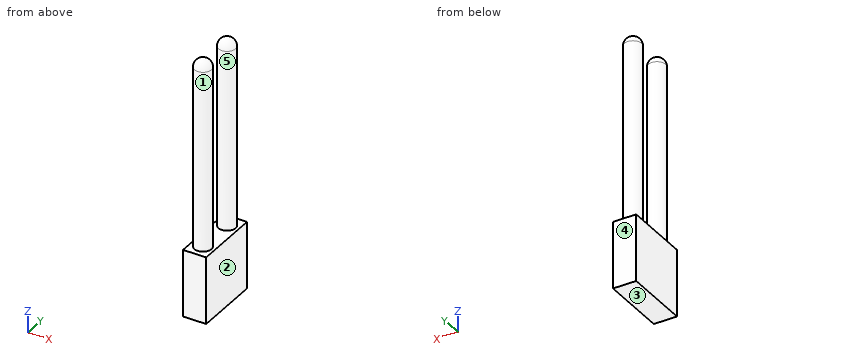
from build123d import *

# Parameters (mm, degrees)
F0_W     = 39
F0_H     = 39
F1_DEPTH = 13.5
F2_R     = 5
F3_DEPTH = 110
F4_R     = 5


with BuildPart() as f1:
    # F0 (on Right) → F1 (new body)
    with BuildSketch(Plane.YZ):
        Rectangle(F0_W, F0_H)
    extrude(amount=F1_DEPTH)

    # F2 (on face) → F3 (join)
    with BuildSketch(Plane.XY.offset(19.5)):
        with Locations((6.75, 11.5)):
            Circle(F2_R)
        with Locations((6.75, -11.5)):
            Circle(F2_R)
    extrude(amount=F3_DEPTH)

    # F4
    f4_edges = [f1.edges().sort_by_distance(p)[0] for p in [
        (1.75, 11.5, 129.5),
        (1.75, -11.5, 129.5),
    ]]
    fillet(f4_edges, radius=F4_R)


solid = f1.part
Design review of the part built by this model. Coordinates are the model's own, in mm. Face numbers are marked on the shaded views. A direction names the side the tool comes from. Round coordinates to 2 decimals unless told otherwise and drop trailing zeros. Loops run counter-clockwise (first coordinate to the right, second up) from the corner with the lowest first, then second, coordinate; pieces in that order, holes last. Notation, with made-up numbers: (-32, 1) -> (-4, 1) arc R5 cw to (-4, 6) -> close; hole circle Ø3 at (-37.5, 66). An arc over 180 degrees is marked (long way). Use one line per item in the form item = value. Start each with the question number.
Q1. Wall thickness on line 1 along Z through (x, y) = (2.5, -16.5); line 2 along X through (y, z) = (-12, 93.5); line 3 along Y through (x, z) = (8.5, 113): over which ranges is each line inside the solid? List them lowest first. Write a range as [from, to].
Q2. Draft analysis for pull direction Y (two halves, no side actions). For the marked faces 3, 4 and 5, state which applies: +Y half, -Y half, draft (parallel to the pull), parting line (faces both ways), or undercut.
Q3. For pin 1 Ø6 at (x, z) = (2.5, 92.5) entering from +Y; pin 2 Ø12 at (y, z) = (-2, 53.5) entering from +X; pin 3 Ø6 at (x, z) = (8.5, 113.5) entering from +Y, all flat-tipped, find the tip position at first contact; note any pin that passes through.
Q4. We need section B-B on z = 53. Give the boundary of the cut face in (x, y).
Q5. We need section C-C on y = -11.5. Give the boundary of the cut face in (x, z).
Q6. Machinability: for the marked faces 1 and 2, which of the approach directions +Z, -Z, +X, -X, +Y, -Y give a long, thin tool a straight path to every point of the face, cutting with its end or side? Answer none if there is none.
Q7. We need section A-A on x = 6.75. Give the boundary of the cut face in (y, z).
Calculated:
q1.line_1 = [-19.5, 19.5]
q1.line_2 = [1.78, 11.72]
q1.line_3 = [-16.18, -6.82], [6.82, 16.18]
q2.face_3 = draft
q2.face_4 = +Y half
q2.face_5 = undercut
q3.pin_1 = 16.34
q3.pin_2 = 10.32
q3.pin_3 = 16.5
q4.outline = circle Ø10 at (6.75, -11.5); circle Ø10 at (6.75, 11.5)
q5.outline = (0, -19.5) -> (13.5, -19.5) -> (13.5, 19.5) -> (11.75, 19.5) -> (11.75, 124.5) arc R5 ccw to (1.75, 124.5) -> (1.75, 19.5) -> (0, 19.5) -> close
q6.face_1 = +Z
q6.face_2 = +Z, -Z, +X, +Y, -Y
q7.outline = (-19.5, -19.5) -> (19.5, -19.5) -> (19.5, 19.5) -> (16.5, 19.5) -> (16.5, 124.5) arc R5 ccw to (6.5, 124.5) -> (6.5, 19.5) -> (-6.5, 19.5) -> (-6.5, 124.5) arc R5 ccw to (-16.5, 124.5) -> (-16.5, 19.5) -> (-19.5, 19.5) -> close
